Build history of the part. All positions in model axes, mm. A direction names the side the tool comes from. Round coordinates to 2 decimals unless told otherwise and drop trailing zeros. Order: outer loops, then holes, each group sorted by start corner. A loop starts at its lowest first (then second) coordinate and runs counter-clockwise, first axis right, second up. Notation, with made-up numbers: (56, 19) - (70, 19) arc R18 ccw to (70, 35) - close; hole circle Ø2 at (63, -10). An arc over 180 degrees is marked (long way). One line per question, with ' | ' between items. Start each with the question number.
from build123d import *

# Parameters (mm, degrees)
SKETCH2_W          = 4
SKETCH2_H          = 4.3
CUT_EXTRUDE1_DEPTH = 83.314543369


with BuildPart() as part:
    # Sketch1 → Revolve1 (revolve)
    with BuildSketch(Plane(origin=(0, 0, 0), x_dir=(0, 0, -1), z_dir=(1, 0, 0)), mode=Mode.PRIVATE) as revolve1_sk:
        Polygon((55.295, -5.75), (55.295, 5.75), (57.295, 5.75), (57.295, 7.25), (6, 7.25), (6, -7.25), (57.295, -7.25), (57.295, -5.75), align=None)
    revolve(revolve1_sk.sketch.rotate(Axis((0, 10.31552251, 0), (0, -1, 0)), 180), axis=Axis((0, 10.31552251, 0), (0, -1, 0)))

    # Sketch2 → Cut-Extrude1 (cut, through all)
    with BuildSketch(Plane(origin=(0, 7.25, 0), x_dir=(1, 0, 0), z_dir=(0, 1, 0))):
        with Locations((0, 5.65)):
            Rectangle(SKETCH2_W, SKETCH2_H)
    extrude(amount=-CUT_EXTRUDE1_DEPTH, mode=Mode.SUBTRACT)


solid = part.part
Item 1: Slice it at C-C (y = -0.75). Write the cut outline in (x, z) (3 decimals), plus the area to 3 significant figures.
Item 2: Slice it at A-A (z = 0). Write the cut outline in (x, y) (3 decimals), plus the area to 3 significant figures.
Item 3: 3-axis set-ups, long thin cutter, end or side, ignore diameter. For faces 1 (the face through (12, -7.25, 1)), 2 (the face through (-47, 5.75, 30)), 3 (the face through (0, 0, -7.8)): which of +Z, -Z, +X, -X, +Y, -Y reach the whole face in a straight line?
Item 4: Pull direction Y, two halves, no side cores. Call faces 4 (the face through (12, 7.25, -1)), 5 (the face through (-54.824, 0.08, -7.198)), 6 (the face through (55.933, 6.51, -12.42)): released by +Y, released by -Y, zero draft, split by the parting line, or undercut.
Item 5: Slice it at D-D (z = -50). Write the cut outline in (x, y).
Item 6: Slice it at B-B (x = 0). Write the cut outline in (y, z) (3 decimals), plus the area to 3 significant figures.
Item 7: Wall check: line 1 along X through (y, z) = (1.75, 0) (3 decimals); line 2 along X through (y, z) = (5, -5); line 3 along Z through (x, y) = (-14, 5.25). Give the ranges that are in metal, low to high. Write a range as [from, to].
Item 8: Pin check, flat tips, straight feed: pin 1 (1 mm diameter, centred on x = 40, y = 3.5, fed in from -Z); pin 2 (1 mm diameter, centred on y = 3, z = -30.5, fed in from -X); pin 3 (5 mm diameter, centred on x = -35, y = -5.5, fed in from +Z). Stop position of each tip, or through.
A:
1) outline: circle Ø110.59 at (0, 0); hole (-2, -7.8) - (2, -7.8) - (2, -5.657) arc R6 ccw (long way) to (-2, -5.657) - close | area: 9,480 mm^2
2) outline: (-57.295, -7.25) - (-6, -7.25) - (-6, 7.25) - (-57.295, 7.25) - (-57.295, 5.75) - (-55.295, 5.75) - (-55.295, -5.75) - (-57.295, -5.75) - close; (6, -7.25) - (57.295, -7.25) - (57.295, -5.75) - (55.295, -5.75) - (55.295, 5.75) - (57.295, 5.75) - (57.295, 7.25) - (6, 7.25) - close | area: 1,440 mm^2
3) face 1: +Z, -Z, +X, -X, -Y | face 2: none | face 3: +Y, -Y
4) face 4: released by +Y | face 5: undercut | face 6: zero draft
5) outline: (-27.98, -7.25) - (27.98, -7.25) - (27.98, -5.75) - (23.61, -5.75) - (23.61, 5.75) - (27.98, 5.75) - (27.98, 7.25) - (-27.98, 7.25) - (-27.98, 5.75) - (-23.61, 5.75) - (-23.61, -5.75) - (-27.98, -5.75) - close
6) outline: (-7.25, -57.295) - (-5.75, -57.295) - (-5.75, -55.295) - (5.75, -55.295) - (5.75, -57.295) - (7.25, -57.295) - (7.25, -7.8) - (-7.25, -7.8) - close; (-7.25, 6) - (7.25, 6) - (7.25, 57.295) - (5.75, 57.295) - (5.75, 55.295) - (-5.75, 55.295) - (-5.75, 57.295) - (-7.25, 57.295) - close | area: 1,420 mm^2
7) line 1: [-55.295, -6], [6, 55.295] | line 2: [-55.07, -3.32], [3.32, 55.07] | line 3: [-53.49, 53.49]
8) pin 1: z = -38.69 | pin 2: x = -46.45 | pin 3: z = 47.18
